Input: part model. Units: mm. Frame: model coordinates. A direction names the side the tool comes from. Coordinates: 2 decimals unless noted, no trailing zeros. Write each loop counter-clockwise with the first axis right and the second up, starting at its lowest first coordinate (ties: lowest second). Pieces come first, ordered by that corner, then holes. Notation, with made-up numbers: (42.5, -22) - (48.5, -22) arc R13 ccw to (48.5, 0) - close; hole circle Ø11 at (-19, -2.5). An arc over 180 degrees is marked (long way). Put each result on its own line as item: value. Start each with the question number.
1. Line query: line 1 (X direction, y = 22, z = 12); line 2 (Z direction, x = -17.9, y = -15); line 3 (Y direction, x = -39.5, z = 9.5). Output: solid intervals per line, ascending.
2. Cut plane D-D, the plane y = -15. Return loops of the section in (x, z).
3. Access query for faces 1 (the cylindrical face through (-19.985, 24.145, 10.14)), 2 (the flat face through (-44.083, 7, 10)), 3 (the flat face through (-43, -20, 10)). Directions: +Z, -Z, +X, -X, +Y, -Y. A direction counts if a zero-diameter tool reaches every point of the face in a straight line with its end or side. Return the directions, or none.
4. Pin query (flat end, axial travel): pin 1 (4.5 mm diameter, centred on y = -15, z = 10, fed in from -X). Return the tip coordinate at first contact, or that it passes through.
5. Cut plane A-A, the plane y = 16. Return loops of the section in (x, z).
6. Cut plane B-B, the plane z = 10. Return loops of the section in (x, y).
7. Cut plane C-C, the plane x = -43. Return loops of the section in (y, z), and give its area (3 significant figures).
8. Pull-direction query (X, two-part tool) for faces 4 (the flat face through (-18, -20, 10)), 5 (the cylindrical face through (-43.228, 24.098, 10.14)), 6 (the cylindrical face through (-45.658, 26.496, 10.14)); classes: released by +X, released by -X, zero draft, split by the parting line, or undercut.
from build123d import *

# Parameters (mm, degrees)
F0_W     = 25
F0_H     = 3
F0_W_2   = 3
F0_H_2   = 20
F1_DEPTH = 20
F3_D     = 4
F3_DEPTH = 120
F4_R     = 3
F5_R     = 5


with BuildPart() as f1:
    # F0 (on Top) → F1 (new body)
    with BuildSketch(Plane.XY):
        Polygon((-44.083337, -10), (-44.083337, 0), (-47.083337, 0), (-47.083337, -20), (-39.083337, -20), (-39.083337, -10), align=None)
        Polygon((-47.083337, 0), (-44.083337, 0), (-44.083337, 25), (-44.083337, 28), (-47.083337, 28), align=None)
        with Locations((-31.583337, 26.5)):
            Rectangle(F0_W, F0_H)
        Polygon((-19.083337, 25), (-19.083337, 0), (-16.083337, 0), (-16.083337, 28), (-19.083337, 28), align=None)
        with Locations((-17.583337, -10)):
            Rectangle(F0_W_2, F0_H_2)
    extrude(amount=F1_DEPTH)

    # F3
    with Locations(Plane(origin=(-47.083337, 0, 0), x_dir=(0, -1, 0), z_dir=(-1, 0, 0))):
        with Locations((15, 10)):
            Hole(F3_D / 2, depth=F3_DEPTH)

    # F4
    f4_edges = [f1.edges().sort_by_distance(p)[0] for p in [
        (-19.083337, 25, 10),
        (-44.083337, 25, 10),
        (-44.083337, -10, 10),
    ]]
    fillet(f4_edges, radius=F4_R)

    # F5
    f5_edges = [f1.edges().sort_by_distance(p)[0] for p in [
        (-47.083337, 28, 10),
        (-16.083337, 28, 10),
    ]]
    fillet(f5_edges, radius=F5_R)


solid = f1.part
Report:
1. line 1: x = -47.08 to -44.08, -19.08 to -16.08
1. line 2: z = 0 to 8, 12 to 20
1. line 3: y = -20 to -16.94, -13.06 to -10, 25 to 28
2. outline: (-47.08, 0) - (-39.08, 0) - (-39.08, 8) - (-47.08, 8) - close; (-47.08, 12) - (-39.08, 12) - (-39.08, 20) - (-47.08, 20) - close; (-19.08, 0) - (-16.08, 0) - (-16.08, 8) - (-19.08, 8) - close; (-19.08, 12) - (-16.08, 12) - (-16.08, 20) - (-19.08, 20) - close
3. face 1: +Z, -Z, -Y
3. face 2: +Z, -Z
3. face 3: +Z, -Z, +X, -X, -Y
4. pin 1: stops at x = -47.08
5. outline: (-47.08, 0) - (-44.08, 0) - (-44.08, 20) - (-47.08, 20) - close; (-19.08, 0) - (-16.08, 0) - (-16.08, 20) - (-19.08, 20) - close
6. outline: (-47.08, -20) - (-39.08, -20) - (-39.08, -17) - (-47.08, -17) - close; (-47.08, -13) - (-39.08, -13) - (-39.08, -10) - (-41.08, -10) arc R3 cw to (-44.08, -7) - (-44.08, 22) arc R3 cw to (-41.08, 25) - (-22.08, 25) arc R3 cw to (-19.08, 22) - (-19.08, -13) - (-16.08, -13) - (-16.08, 23) arc R5 ccw to (-21.08, 28) - (-42.08, 28) arc R5 ccw to (-47.08, 23) - close; (-19.08, -20) - (-16.08, -20) - (-16.08, -17) - (-19.08, -17) - close
7. outline: (-20, 0) - (-9.31, 0) - (-9.31, 20) - (-20, 20) - close; (24.31, 0) - (27.92, 0) - (27.92, 20) - (24.31, 20) - close; hole circle Ø4 at (-15, 10)
7. area: 273 mm^2
8. face 4: zero draft
8. face 5: undercut
8. face 6: released by -X
